CAD build for the part. Positions are in the model's coordinates, mm. A direction names the side the tool comes from. Round coordinates to 2 decimals unless told otherwise and drop trailing zeros. Order: outer loops, then holes, each group sorted by start corner. A loop starts at its lowest first (then second) coordinate and runs counter-clockwise, first axis right, second up. Notation, with made-up numbers: (18, 31) - (66, 31) arc R14 ccw to (66, 46) - close; hole circle Ø8 at (80, 32). An arc over 180 degrees is marked (long way). Use one line per item in the form item = value. Start each with the question number.
Autodesk Inventor part; units mm, degrees
ref_plane "YZ Plane" through (0, 0, 0) normal (1, 0, 0) x (0, 1, 0)
ref_plane "XZ Plane" through (0, 0, 0) normal (0, 1, 0) x (-1, 0, 0)
ref_plane "XY Plane" through (0, 0, 0) normal (0, 0, 1) x (1, 0, 0)
sketch "Sketch1" plane through (0, 0, 0) normal (1, 0, 0) x (0, 1, 0)
  arc A0 (-24.3967, 0) -> (-49.3967, -25) centre (-24.3967, -25) ccw
  line L0 (-10.5765, 0) -> (-24.3967, 0)
  line L1 (-10.5765, 0) -> (63.7352, 0)
  line L2 (-24.3967, 0) -> (-39.3967, 0)
  line L3 (-39.3967, 0) -> (-39.3967, -5)
  line L4 (-39.3967, 0) -> (-3.4641, 0)
  line L5 (0, 4) -> (-39.3967, 4)
  line L6 (-39.3967, 4) -> (-39.3967, 0)
  line L7 (0, 4) -> (20, 4)
  line L8 (20, 4) -> (20, 0)
  line L9 (-3.4641, 0) -> (20, 0)
  point P0 (0, 0)
  dimension "d0" = 15
  dimension "d8" = 20
  dimension "d12" = 4
extrude "Extrusion1" add sketch "Sketch1" along normal mid plane 20
sketch "Sketch4" plane through (-10, 20, 4) normal (0, 1, 0) x (1, 0, 0)
  line L0 (4.1911, -3.9481) -> (14.8671, -3.9481)
  line L1 (14.8671, -6.4881) -> (4.1911, -6.4881)
  line L2 (0, 0) -> (20, 0)
  line L3 (-12.5359, -24.54) -> (31.5941, -24.54)
  line L4 (34.7691, 0) -> (-15.7109, 0)
  line L5 (-15.7109, 0) -> (34.7691, 0)
  line L6 (3.9411, -6.2381) -> (3.9411, -4.1981)
  arc A0 (3.9411, -6.2381) -> (4.1911, -6.4881) centre (4.1911, -6.2381) ccw
  arc A1 (4.1911, -3.9481) -> (3.9411, -4.1981) centre (4.1911, -4.1981) ccw
  line L7 (0, 4) -> (0, 0)
  circle A2 centre (-3.4709, -13.9481) radius 8.5
  arc A3 (-15.7109, -21.365) -> (-12.5359, -24.54) centre (-12.5359, -21.365) ccw
  line L8 (-15.7109, -21.365) -> (-15.7109, 0)
  arc A4 (31.5941, -24.54) -> (34.7691, -21.365) centre (31.5941, -21.365) ccw
  line L9 (34.7691, 0) -> (34.7691, -21.365)
  line L10 (20, 0) -> (20, 4)
  line L11 (20, 4) -> (20, 2)
  arc A5 (14.8671, -6.4881) -> (15.1171, -6.2381) centre (14.8671, -6.2381) ccw
  arc A6 (15.1171, -4.1981) -> (14.8671, -3.9481) centre (14.8671, -4.1981) ccw
  circle A7 centre (22.5291, -13.9481) radius 8.5
  line L12 (15.1171, -4.1981) -> (15.1171, -6.2381)
  line L13 (0, 2) -> (0, 0)
  line L14 (0, 0) -> (20, 0)
  line L15 (20, 0) -> (20, 2)
  line L16 (0, 0) -> (20, 0)
  line L17 (20, 4) -> (20, 0)
  line L18 (20, 4) -> (0, 4)
  line L19 (0, 0) -> (0, 4)
  point P0 (10, 4)
  point P1 (10, 2)
  point P2 (10, 4)
  point P3 (10, 0)
  point P4 (10, 0)
  point P5 (24.7691, -1.4081)
  point P6 (10, 4)
  dimension "d9" = 4
extrude "Extrusion3" add sketch "Sketch4" along normal blind 3
properties part number "SensorMount"
(1) Flat gauge pins, fed straight in: P1, Ø6, axis at x = 0.5, y = -16, coming from the +Z side; P2, Ø10, axis at x = 3.5, y = -11, coming from the -Z side; P3, Ø7, axis at y = -10.5, z = -2.5, coming from the -X side. Where does each tip first touch, or does it go through?
(2) Slice it at A-A (x = -16). Give the cut face in (y, z).
(3) Slice it at B-B (z = 13.5). Give the cut face in (x, y).
(4) Which spindle directions (+Z, -Z, +X, -X, +Y, -Y) get a long thin tool onto all of the face, cutting with end or side? Do faces 4 (the flat face through (-1, 20, 16)), 5 (the flat face through (0, -1, 0)), 6 (the flat face through (5.117, 21, 9)). Say none if no direction does.
(5) Slice it at C-C (y = -16.5). Give the cut face in (x, z), and give its area (3 significant figures).
(6) Mould opens along Z. For faces 1 (the cylindrical face through (23.86, 21.48, 27.59)), 2 (the cylindrical face through (-5.363, 21.479, 20.501)), 3 (the flat face through (-25.711, 21, 15)) say: pulls with the +Z half, pulls with the -Z half, needs draft (parallel to the pull), parting line crosses it, or undercut.
(7) Slice it at D-D (z = 20.5). Give the cut face in (x, y).
(8) Wall check: line 1 (Y direction, x = -23, z = 25.5); line 2 (Z direction, x = 8.5, y = 16); line 3 (X direction, y = -17.5, z = 3). Give the ranges that are in metal, low to high. Write a range as [from, to].
Results list:
q1.P1 = 4
q1.P2 = 0
q1.P3 = -10
q2.outline = (20, 4) - (23, 4) - (23, 9.83) - (20, 9.83) - close; (20, 26.06) - (23, 26.06) - (23, 28.54) - (20, 28.54) - close
q3.outline = (-25.71, 20) - (-20.71, 20) - (-20.71, 23) - (-25.71, 23) - close; (-6.23, 20) - (5.29, 20) - (5.29, 23) - (-6.23, 23) - close; (19.77, 20) - (24.77, 20) - (24.77, 23) - (19.77, 23) - close
q4.face_4 = +Z, +X, -X, -Y
q4.face_5 = -Z, +X, -X, +Y
q4.face_6 = +Y, -Y
q5.outline = (-10, 0) - (10, 0) - (10, 4) - (-10, 4) - close
q5.area = 80.0 mm²
q6.face_1 = pulls with the +Z half
q6.face_2 = undercut
q6.face_3 = needs draft
q7.outline = (-25.71, 20) - (-21.58, 20) - (-21.58, 23) - (-25.71, 23) - close; (-5.36, 20) - (4.42, 20) - (4.42, 23) - (-5.36, 23) - close; (20.64, 20) - (24.77, 20) - (24.77, 23) - (20.64, 23) - close
q8.line_1 = [20, 23]
q8.line_2 = [0, 4]
q8.line_3 = [-10, 10]
